from build123d import *

# Parameters (mm, degrees)
F0_R     = 0.40005
F1_DEPTH = 6.4262
F2_R     = 0.99695
F2_R_2   = 0.40005
F3_DEPTH = 0.7493
F4_R     = 3.5052
F4_R_2   = 0.99695
F5_DEPTH = 16.6243
F6_R     = 0.92075
F7_DEPTH = 0.9525


with BuildPart() as f1:
    # F0 (on Front) → F1 (new body)
    with BuildSketch(Plane.XZ):
        Circle(F0_R)
    extrude(amount=-F1_DEPTH)

    # F2 (on face) → F3 (join)
    with BuildSketch(Plane(origin=(0, 6.4262, 0), x_dir=(-1, 0, 0), z_dir=(0, 1, 0))):
        Circle(F2_R)
        Circle(F2_R_2, mode=Mode.SUBTRACT)
        Circle(F2_R_2)
    extrude(amount=F3_DEPTH)

    # F4 (on face) → F5 (join)
    with BuildSketch(Plane(origin=(0, 7.1755, 0), x_dir=(-1, 0, 0), z_dir=(0, 1, 0))):
        Circle(F4_R)
        Circle(F4_R_2, mode=Mode.SUBTRACT)
        Circle(F4_R_2)
    extrude(amount=F5_DEPTH)

    # F6 (on face) → F7 (join)
    with BuildSketch(Plane(origin=(0, 23.7998, 0), x_dir=(-1, 0, 0), z_dir=(0, 1, 0))):
        Circle(F6_R)
    extrude(amount=F7_DEPTH)


solid = f1.part
Input: part model. Units: mm. Frame: model coordinates. A direction names the side the tool comes from. Coordinates: 2 decimals unless noted, no trailing zeros. Write each loop counter-clockwise with the first axis right and the second up, starting at its lowest first coordinate (ties: lowest second). Pieces come first, ordered by that corner, then holes. Notation, with made-up numbers: M 38,-15.75 L 51,-15.75 A18 cw 51,-2.75 Z; hole C 40.5,53.5 d9. An arc over 180 degrees is marked long. Answer as a JSON object with one key per item and string values. Group by question number.
(1) Set-up query: faces 1 (the face through (-3.343, 15.371, 1.053)), 2 (the face through (-0.95, 6.8, 0.3)), 3 (the face through (-0.42, 24.27, -0.82)). Return all of +Z, -Z, +X, -X, +Y, -Y with unobstructed straight access to the full face (end or side cutting, diameter ignored); none if empty.
(2) Section B-B on x = 0. Output: boundary loops of the cut face in (y, z).
(3) Contact query for flat-ended pins moving along their axis: P1, Ø3.5, axis at x = -1.5, z = 0, coming from the +Y side; P2, Ø2, axis at x = 2.5, z = -2, coming from the +Y side; P3, Ø1.5, axis at y = 13, z = -1, coming from the -X side. Output: stop coordinate, or through.
(4) Section A-A on z = 0. Output: boundary loops of the cut face in (x, y), plus the area to 3 significant figures.
(5) Ray query, line 1 along Y through (x, z) = (1, 2.25); line 2 along Y through (x, z) = (0, -0.5); line 3 along X through (y, z) = (22.5, -1). Return the intervals inside material, ascending. Write a range as [from, to].
(6) Section C-C on y = 8.25. Output: boundary loops of the cut face in (x, z).
(7) Section D-D on z = -2. Output: boundary loops of the cut face in (x, y), plus the area to 3 significant figures.
Result set:
{
 "1": {"face 1": "+Y, -Y", "face 2": "-Y", "face 3": "+Y"},
 "2": {"outline": "M 0,-0.4 L 6.43,-0.4 L 6.43,-1 L 7.18,-1 L 7.18,-3.51 L 23.8,-3.51 L 23.8,-0.92 L 24.75,-0.92 L 24.75,0.92 L 23.8,0.92 L 23.8,3.51 L 7.18,3.51 L 7.18,1 L 6.43,1 L 6.43,0.4 L 0,0.4 Z"},
 "3": {"P1": "stops at y = 24.75", "P2": "stops at y = 23.8", "P3": "stops at x = -3.5"},
 "4": {"outline": "M -3.51,7.18 L -1,7.18 L -1,6.43 L -0.4,6.43 L -0.4,0 L 0.4,0 L 0.4,6.43 L 1,6.43 L 1,7.18 L 3.51,7.18 L 3.51,23.8 L 0.92,23.8 L 0.92,24.75 L -0.92,24.75 L -0.92,23.8 L -3.51,23.8 Z", "area": "125 mm2"},
 "5": {"line 1": "y = [7.18, 23.8]", "line 2": "y = [6.43, 24.75]", "line 3": "x = [-3.36, 3.36]"},
 "6": {"outline": "C 0,0 d7.01"},
 "7": {"outline": "M -2.88,7.18 L 2.88,7.18 L 2.88,23.8 L -2.88,23.8 Z", "area": "95.7 mm2"}
}
